Verification items for this drawing (mm, ordinates from the low corner). Round coordinates to 2 decimals unless told otherwise and drop trailing zeros. Write each loop counter-clockwise with the first axis right and the second up, starting at its lowest first coordinate (ties: lowest second). Pieces come first, ordered by that corner, then holes.
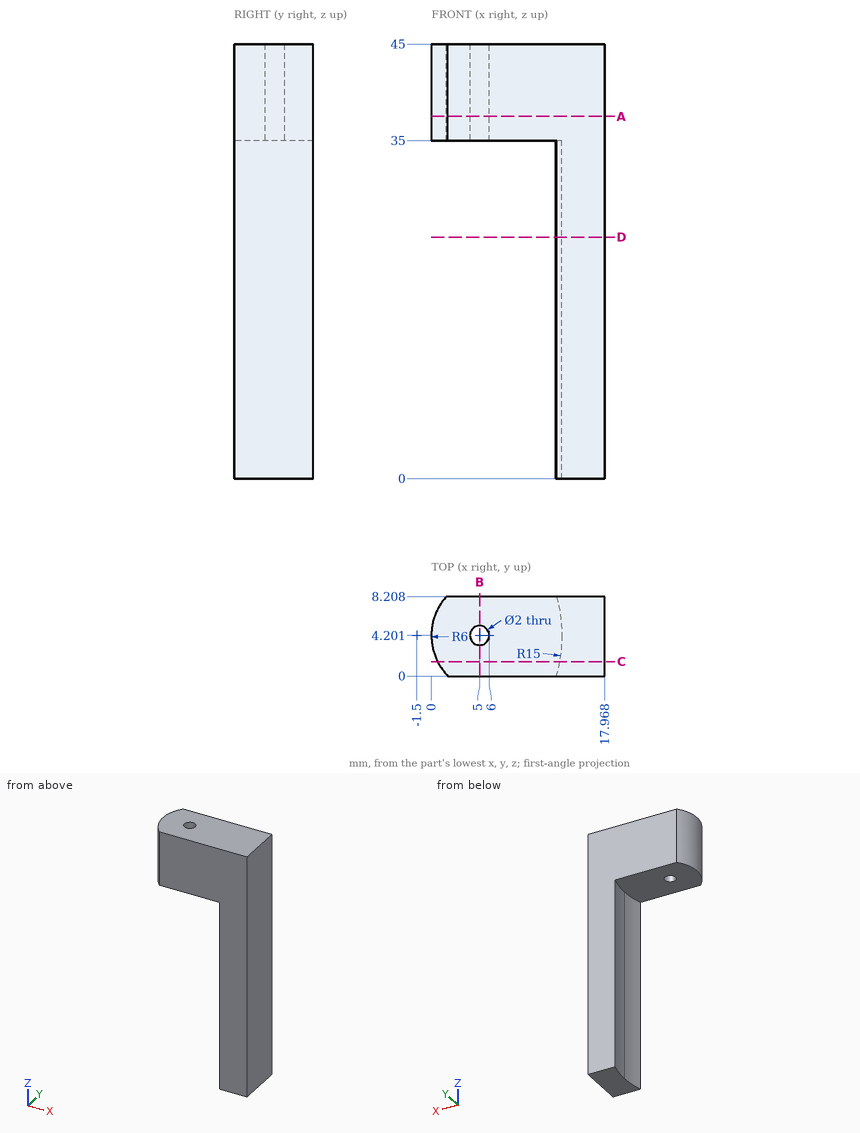
1. Section check A-A (z = 37.5). Record the cut outline in (x, y) (1 decimal), plus the area to 3 significant figures.
2. Depth check by flat-ended pin: pin 1 Ø2.5 at (x, y) = (5, 4.2) entering from -Z; pin 2 Ø1 at (y, z) = (5.5, 15.5) entering from -X. Enter the tip coordinate at first touch or a pass-through.
3. Section check C-C (y = 1.5). Record the cut outline in (x, z) (1 decimal), plus the area to 3 significant figures.
4. Scan lines: line 1 along Y through (x, z) = (5, 41.5); line 2 along Z through (x, y) = (7.25, 3.25); line 3 along X through (y, z) = (4.5, 21.5). Record each from-to range of solid material in increasing order.
5. Section check B-B (x = 5). Record the cut outline in (y, z).
6. Section check D-D (z = 25). Record the cut outline in (x, y) (1 decimal).
Results below:
1. outline: (1.5, 8.2) arc R6 ccw to (1.7, 0) - (18, 0) - (18, 8.2) - close; hole circle Ø2 at (5, 4.2)
1. area: 140 mm2
2. pin 1: stops at z = 35
2. pin 2: stops at x = 13.39
3. outline: (0.6, 35) - (13.3, 35) - (13.3, 0) - (18, 0) - (18, 45) - (0.6, 45) - close
3. area: 338 mm2
4. line 1: y = 0 to 3.2, 5.2 to 8.21
4. line 2: z = 35 to 45
4. line 3: x = 13.5 to 17.97
5. outline: (0, 35) - (3.2, 35) - (3.2, 45) - (0, 45) - close; (5.2, 35) - (8.21, 35) - (8.21, 45) - (5.2, 45) - close
6. outline: (12.9, 0) - (18, 0) - (18, 8.2) - (13, 8.2) arc R15 cw to start
